```python
from build123d import *

# Parameters (mm, degrees)
SKETCH1_W           = 615.95
SKETCH1_H           = 203.2
BOSS_EXTRUDE1_DEPTH = 3.175
SKETCH2_W           = 152.4
SKETCH2_H           = 127
CUT_EXTRUDE1_DEPTH  = 325.316575663
SKETCH3_W           = 6.35
SKETCH3_H           = 25.4
CUT_EXTRUDE2_DEPTH  = 325.316575663
SKETCH4_R           = 1.75
CUT_EXTRUDE3_DEPTH  = 325.316575663
SKETCH5_W           = 62.23
SKETCH5_H           = 29.21
CUT_EXTRUDE4_DEPTH  = 325.316575663


with BuildPart() as part:
    # Sketch1 → Boss-Extrude1 (new body)
    with BuildSketch(Plane.XY):
        Rectangle(SKETCH1_W, SKETCH1_H)
    extrude(amount=BOSS_EXTRUDE1_DEPTH)

    # Sketch2 → Cut-Extrude1 (cut, through all)
    with BuildSketch(Plane.XY.offset(3.175)):
        with Locations((-193.675, 0)):
            Rectangle(SKETCH2_W, SKETCH2_H)
    extrude(amount=-CUT_EXTRUDE1_DEPTH, mode=Mode.SUBTRACT)

    # Sketch3 → Cut-Extrude2 (cut, through all)
    with BuildSketch(Plane.XY.offset(3.175)):
        with Locations((-15.875, 25.4)):
            Rectangle(SKETCH3_W, SKETCH3_H)
    extrude(amount=-CUT_EXTRUDE2_DEPTH, mode=Mode.SUBTRACT)

    # Sketch4 → Cut-Extrude3 (cut, through all)
    with BuildSketch(Plane.XY.offset(3.175)):
        with Locations((0.635, 31.75)):
            Circle(SKETCH4_R)
        with Locations(Location((-32.385, 31.75, 0), (0, 0, 180))):
            Circle(SKETCH4_R)
    extrude(amount=-CUT_EXTRUDE3_DEPTH, mode=Mode.SUBTRACT)

    # Sketch5 → Cut-Extrude4 (cut, through all)
    with BuildSketch(Plane.XY.offset(3.175)):
        with Locations((-15.875, -48.895)):
            Rectangle(SKETCH5_W, SKETCH5_H)
    extrude(amount=-CUT_EXTRUDE4_DEPTH, mode=Mode.SUBTRACT)


solid = part.part
```
Can you work these out from the model? Positions are in its coordinate system, mm. Give positions to 0.01 mm unless a question says otherwise; leave off trailing zeros. Loops run counter-clockwise (first coordinate to the right, second up) from the corner with the lowest first, then second, coordinate; pieces in that order, holes last. Notation, with made-up numbers: M 4.25,79 L 38.25,79 A23 ccw 38.25,114 Z; hole C 78,13 d5. An arc over 180 degrees is marked long. Use CSV: the item, a comma, the result in double quotes. Start each with the question number.
1. Imagine slicing it at B-B, the plane x = -187. Write out the boundary of the cut face in (y, z) (3 decimals).
2. Imagine slicing it at D-D, the plane y = 22.5. Write out the boundary of the cut face in (x, z) (3 decimals), plus the area to 3 significant figures.
3. Imagine slicing it at A-A, the plane y = -16.5. Write out the boundary of the cut face in (x, z) (3 decimals).
4. Imagine slicing it at C-C, the plane z = 2. Write out the boundary of the cut face in (x, y) (3 decimals).
5. If I drill on L1, parallel to X at y = 27.5, z = 0.4 (3 decimals); L2, parallel to Y at x = -33, z = 0.7; L3, parallel to X at y = -57.5, z = 0.7 (3 decimals), over which ranges is the centre line in solid material (lowest first)?
6. For P1, Ø2, axis at x = 242.5, y = 29, coming from the -Z side, with a flat end and sliding along its axis, tell me the tip position at first contact or that it passes through.
Response values:
1,outline,"M -101.6,0 L -63.5,0 L -63.5,3.175 L -101.6,3.175 Z; M 63.5,0 L 101.6,0 L 101.6,3.175 L 63.5,3.175 Z"
2,outline,"M -307.975,0 L -269.875,0 L -269.875,3.175 L -307.975,3.175 Z; M -117.475,0 L -19.05,0 L -19.05,3.175 L -117.475,3.175 Z; M -12.7,0 L 307.975,0 L 307.975,3.175 L -12.7,3.175 Z"
2,area,"1,450 mm^2"
3,outline,"M -307.975,0 L -269.875,0 L -269.875,3.175 L -307.975,3.175 Z; M -117.475,0 L 307.975,0 L 307.975,3.175 L -117.475,3.175 Z"
4,outline,"M -307.975,-101.6 L 307.975,-101.6 L 307.975,101.6 L -307.975,101.6 Z; hole M -269.875,-63.5 L -117.475,-63.5 L -117.475,63.5 L -269.875,63.5 Z; hole M -46.99,-63.5 L 15.24,-63.5 L 15.24,-34.29 L -46.99,-34.29 Z; hole C -32.385,31.75 d3.5; hole M -19.05,12.7 L -12.7,12.7 L -12.7,38.1 L -19.05,38.1 Z; hole C 0.635,31.75 d3.5"
5,L1,"-307.975 to -269.875, -117.475 to -19.05, -12.7 to 307.975"
5,L2,"-101.6 to -63.5, -34.29 to 30.11, 33.39 to 101.6"
5,L3,"-307.975 to -269.875, -117.475 to -46.99, 15.24 to 307.975"
6,P1,"z = 0"
